For this review, take the finished solid that the model builds, in its own axes (mm). Face numbers are marked on the shaded views. A direction names the side the tool comes from. Coordinates: 2 decimals unless noted, no trailing zeros. Loops run counter-clockwise (first coordinate to the right, second up) from the corner with the lowest first, then second, coordinate; pieces in that order, holes last. Notation, with made-up numbers: M 33,17 L 68,17 A30 ccw 68,50 Z; hole C -38.75,-26 d4. An arc over 180 degrees is marked long. Write item = value, one per line.
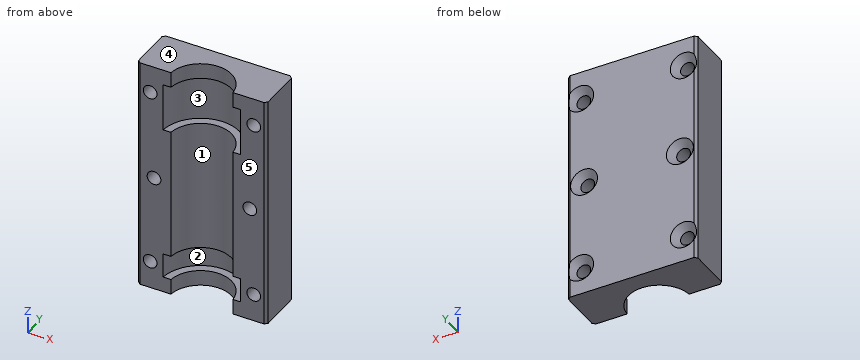
from build123d import *

# Parameters (mm, degrees)
BOSS_EXTRUDE1_DEPTH         = 91
CHAMFER1_SIZE               = 1
SKETCH2_W                   = 6.524852915
SKETCH2_H                   = 18.5
SKETCH2_W_2                 = 5.135295392
SKETCH2_H_2                 = 9.5
HOLE_WIZARD_M51_D           = 5.3
HOLE_WIZARD_M51_CSINK_D     = 10.4
HOLE_WIZARD_M51_CSINK_ANGLE = 90


with BuildPart() as part:
    # Sketch1 → Boss-Extrude1 (new body)
    with BuildSketch(Plane.XY):
        with BuildLine():
            Line((11.958260743, 1), (25, 1))
            Line((25, 1), (25, 19))
            Line((25, 19), (-25, 19))
            Line((-25, 19), (-25, 1))
            Line((-25, 1), (-11.958260743, 1))
            ThreePointArc((-11.958260743, 1), (0, 12), (11.958260743, 1))
        make_face()
    extrude(amount=-BOSS_EXTRUDE1_DEPTH)

    # Chamfer1
    chamfer1_edges = [part.edges().sort_by_distance(p)[0] for p in [
        (-25, 19, -45.5),
        (25, 19, -45.5),
        (25, 1, -45.5),
        (-25, 1, -45.5),
    ]]
    chamfer(chamfer1_edges, length=CHAMFER1_SIZE)

    # Sketch2 → Cut-Revolve2 (revolve, cut)
    with BuildSketch(Plane.XZ):
        with Locations((11.737573543, -15.25)):
            Rectangle(SKETCH2_W, SKETCH2_H)
        with Locations((12.432352304, -80.25)):
            Rectangle(SKETCH2_W_2, SKETCH2_H_2)
    revolve(axis=Axis((0, 0, 0), (0, 0, -1)), mode=Mode.SUBTRACT)

    # Зенковка для  винта с плоской головкой M51 (through all)
    with Locations(Plane(origin=(0, 19, 0), x_dir=(1, 0, 0), z_dir=(0, 1, 0))):
        with Locations((-20, 80.25), (20, 80.25), (18.5, 45.5), (-18.5, 45.5), (-20, 10.75), (20, 10.75)):
            CounterSinkHole(HOLE_WIZARD_M51_D / 2, HOLE_WIZARD_M51_CSINK_D / 2, counter_sink_angle=HOLE_WIZARD_M51_CSINK_ANGLE)


solid = part.part
Q1. Add section B-B (y = 7). State how many separate pieces and enclosed holes the cut face has, and give its area (3 significant figures).
Solved:
separate_pieces = 2
enclosed_holes = 6
area = 2,450 mm²
Q2. Add section C-C (z = -39). Write out the cut boundary in (x, y), and give its area (3 significant figures).
Solved:
outline = M -25,2 L -24,1 L -11.96,1 A12 cw 11.96,1 L 24,1 L 25,2 L 25,18 L 24,19 L -24,19 L -25,18 Z
area = 696 mm²
Q3. Add section A-A (z = -80.25). Write out the cut boundary in (x, y), and give its area (3 significant figures).
Solved:
outline = M -25,2 L -24,1 L -22.65,1 L -22.65,16.45 L -24.6,18.4 L -25,18 Z; M -17.35,1 L -14.97,1 A15 cw 14.97,1 L 17.35,1 L 17.35,16.45 L 14.8,19 L -14.8,19 L -17.35,16.45 Z; M 22.65,1 L 24,1 L 25,2 L 25,18 L 24.6,18.4 L 22.65,16.45 Z
area = 371 mm²
Q4. For pin 1 Ø4 at (x, z) = (20, -10.75) entering from +Y; pin 2 Ø7 at (x, z) = (-18.5, -45.5) entering from +Y, all flat-tipped, find the tip position at first contact; note any pin that passes through.
Solved:
pin_1 = through
pin_2 = 17.3
Q5. Draft analysis for pull direction Z (two halves, no side actions). For the marked faces 3, 4 and 5, state which applies: +Z half, -Z half, draft (parallel to the pull), parting line (faces both ways), or undercut.
Solved:
face_3 = undercut
face_4 = +Z half
face_5 = draft
Q6. For line 1 along Z through (x, y) = (-5.5, 13.75); line 2 along Z through (x, y) = (20.5, 2.25); line 3 along Z through (x, y) = (-18.5, 9.75), list the stretches that pass through material, from the lowest coordinate up.
Solved:
line_1 = -91 to -85, -75.5 to -24.5, -6 to 0
line_2 = -91 to -82.85, -77.65 to -47.24, -43.76 to -13.35, -8.15 to 0
line_3 = -91 to -82.43, -78.07 to -48.15, -42.85 to -12.93, -8.57 to 0
Q7. Machinability: for the marked faces 1 and 2, which of the approach directions +Z, -Z, +X, -X, +Y, -Y give a long, thin tool a straight path to every point of the face, cutting with its end or side? Answer none if there is none.
Solved:
face_1 = +Z, -Z, -Y
face_2 = -Y
